Part model, mm, in its own coordinate system. A direction names the side the tool comes from. Round coordinates to 2 decimals unless told otherwise and drop trailing zeros. Order: outer loops, then holes, each group sorted by start corner. A loop starts at its lowest first (then second) coordinate and runs counter-clockwise, first axis right, second up. Notation, with made-up numbers: (9, 25) - (26, 25) arc R25 cw to (26, 43) - close; hole circle Ø4 at (70.25, 24). An arc over 180 degrees is marked (long way). Return JSON: item names as keys, results as strings. Group by question number.
Item 1: Saw through at B-B on y = 43. List the corners of the cut face in (x, z), and give its area (3 significant figures).
Item 2: Two-plate mould, pull along X, no slides. Class faces 5 (the face through (-46.04, 1.3, -17.45)), 6 (the face through (11, -11, -35)), 7 (the face through (-14.012, -41.154, -17.451)): released by +X, released by -X, zero draft, split by the parting line, or undercut.
Item 3: Probe probe 1 along Y at (x, z) = (-40, 17); probe 2 along X at (y, z) = (-5, -20.5); probe 3 along Y at (x, z) = (0, 1.5). List the from-to ranges inside material, lowest first.
Item 4: Saw through at D-D on z = 24.5. List the corners of the cut face in (x, y), and give its area (3 significant figures).
Item 5: Saw through at A-A on x = -40. List the corners of the cut face in (y, z), and give its area (3 significant figures).
Item 6: Drop flat-ended pins along their axis: pin 1 (6 mm diameter, centred on x = 152.5, z = 16, fed in from -Y); pin 2 (8 mm diameter, centred on x = -1, z = -0.5, fed in from +Y); pin 3 (13 mm diameter, centred on x = 15, y = -43, fed in from -Z); pin 4 (1.5 mm diameter, centred on x = 29.5, y = 2.5, fed in from +Z). Give the stop position or say it passes through.
Item 7: Tool access for faces 1 (the face through (-25, 9, 14)), 2 (the face through (226, 0, -6)), 3 (the face through (102.63, -9.45, 15.3)), 4 (the face through (102.185, 9.451, -15.413)): list every direction of +Z, -Z, +X, -X, +Y, -Y with a clear straight run to the whole face (end or side of a thin tool).
Item 8: Saw through at C-C on x = 250. List the corners of the cut face in (y, z).
```python
from build123d import *

# Parameters (mm, degrees)
SKETCH1_R           = 25.416099274
SKETCH1_R_2         = 15.345879333
BOSS_EXTRUDE3_DEPTH = 35
BOSS_EXTRUDE4_DEPTH = 21
CUT_EXTRUDE1_DEPTH  = 21
SKETCH1_7_R         = 17.5
SKETCH1_7_R_2       = 12
BOSS_EXTRUDE5_DEPTH = 21
BOSS_EXTRUDE6_START = 14
SKETCH1_8_R         = 5
BOSS_EXTRUDE6_DEPTH = 7
CUT_EXTRUDE2_DEPTH  = 18.5


with BuildPart() as part:
    # Sketch1 → Boss-Extrude3 (new body, symmetric)
    with BuildSketch(Plane.XY):
        Circle(SKETCH1_R)
        Circle(SKETCH1_R_2, mode=Mode.SUBTRACT)
    extrude(amount=BOSS_EXTRUDE3_DEPTH, both=True)

    # Sketch1<6> → Boss-Extrude4 (add, symmetric)
    with BuildSketch(Plane.XY):
        with BuildLine():
            ThreePointArc((234.99166898, -9), (232.5, 0), (234.99166898, 9))
            Line((234.99166898, 9), (87, 13))
            ThreePointArc((87, 13), (86.400314561, 13.01370903), (85.800764144, 13.032413604))
            Line((85.800764144, 13.032413604), (20.667586541, 14.792868853))
            ThreePointArc((20.667586541, 14.792868853), (24.199871215, 7.768161657), (25.416099274, 0))
            ThreePointArc((25.416099274, 0), (24.199871215, -7.768161657), (20.667586541, -14.792868853))
            Line((20.667586541, -14.792868853), (85.800764144, -13.032413604))
            ThreePointArc((85.800764144, -13.032413604), (86.400314561, -13.01370903), (87, -13))
            Line((87, -13), (234.99166898, -9))
        make_face()
    extrude(amount=BOSS_EXTRUDE4_DEPTH, both=True)

    # Sketch2 → Cut-Extrude1 (cut, symmetric)
    with BuildSketch(Plane(origin=(0, 0, 0), x_dir=(1, 0, 0), z_dir=(0, 1, 0))):
        with BuildLine():
            Line((118.656620919, 13.062509397), (234.99166898, 9))
            Line((234.99166898, 9), (234.99166898, 21))
            Line((234.99166898, 21), (87, 21))
            ThreePointArc((87, 21), (102.408517533, 15.35701958), (118.656620919, 13.062509397))
        make_face()
        with BuildLine():
            Line((87, -21), (234.99166898, -21))
            Line((234.99166898, -21), (234.99166898, -9))
            Line((234.99166898, -9), (118.656620919, -13.062509397))
            ThreePointArc((118.656620919, -13.062509397), (102.408517533, -15.35701958), (87, -21))
        make_face()
    extrude(amount=CUT_EXTRUDE1_DEPTH, both=True, mode=Mode.SUBTRACT)

    # Sketch1<7> → Boss-Extrude5 (add, symmetric)
    with BuildSketch(Plane.XY):
        with Locations((250, 0)):
            Circle(SKETCH1_7_R)
        with Locations((250, 0)):
            Circle(SKETCH1_7_R_2, mode=Mode.SUBTRACT)
    extrude(amount=BOSS_EXTRUDE5_DEPTH, both=True)

    # Sketch1<8> → Boss-Extrude6 (add)
    with BuildSketch(Plane.XY.offset(BOSS_EXTRUDE6_START)):
        with BuildLine():
            Line((20.667586541, 14.792868853), (85.800764144, 13.032413604))
            ThreePointArc((85.800764144, 13.032413604), (52.537254482, 22.523369258), (27.53882285, 46.431897657))
            ThreePointArc((27.53882285, 46.431897657), (18.775996279, 55.439527809), (6.484634563, 52.82285862))
            ThreePointArc((6.484634563, 52.82285862), (-13.863951623, 42.202436765), (-36.520978816, 38.525829777))
            ThreePointArc((-36.520978816, 38.525829777), (-51.292032009, 32.441274184), (-49.011059213, 16.629791258))
            ThreePointArc((-49.011059213, 16.629791258), (-46.024075038, 1.080135069), (-46.508202044, -14.746409188))
            ThreePointArc((-46.508202044, -14.746409188), (-51.333950201, -32.367226465), (-33.774741186, -37.412543656))
            ThreePointArc((-33.774741186, -37.412543656), (-13.740515927, -41.247010721), (4.414359967, -50.546139748))
            ThreePointArc((4.414359967, -50.546139748), (17.277164415, -55.799004736), (27.53882285, -46.431897657))
            ThreePointArc((27.53882285, -46.431897657), (52.537254482, -22.523369258), (85.800764144, -13.032413604))
            Line((85.800764144, -13.032413604), (20.667586541, -14.792868853))
            ThreePointArc((20.667586541, -14.792868853), (-25.416099274, 0), (20.667586541, 14.792868853))
        make_face()
        with Locations((15, -43)):
            Circle(SKETCH1_8_R, mode=Mode.SUBTRACT)
        with Locations((-40, -26)):
            Circle(SKETCH1_8_R, mode=Mode.SUBTRACT)
        with Locations((-40, 26)):
            Circle(SKETCH1_8_R, mode=Mode.SUBTRACT)
        with Locations((15, 43)):
            Circle(SKETCH1_8_R, mode=Mode.SUBTRACT)
    boss_extrude6 = extrude(amount=BOSS_EXTRUDE6_DEPTH)

    # Mirror1: Boss-Extrude6 across plane
    add(boss_extrude6.mirror(Plane.XY))

    # Sketch3 → Cut-Extrude2 (cut)
    with BuildSketch(Plane.XY.offset(21)):
        with BuildLine():
            Line((70, 6), (220, 6))
            ThreePointArc((220, 6), (226, 0), (220, -6))
            Line((220, -6), (70, -6))
            ThreePointArc((70, -6), (64, 0), (70, 6))
        make_face()
    cut_extrude2 = extrude(amount=-CUT_EXTRUDE2_DEPTH, mode=Mode.SUBTRACT)

    # Mirror2: Cut-Extrude2 across plane
    add(cut_extrude2.mirror(Plane.XY), mode=Mode.SUBTRACT)


solid = part.part
```
Filled in:
{
 "1": {"outline": "(-11.59, -21) - (10, -21) - (10, -14) - (-11.59, -14) - close; (-11.59, 14) - (10, 14) - (10, 21) - (-11.59, 21) - close; (20, -21) - (29.86, -21) - (29.86, -14) - (20, -14) - close; (20, 14) - (29.86, 14) - (29.86, 21) - (20, 21) - close", "area": "440 mm^2"},
 "2": {"face 5": "released by -X", "face 6": "zero draft", "face 7": "undercut"},
 "3": {"probe 1": "y = -39 to -31, -21 to 21, 31 to 39", "probe 2": "x = -45.8 to -14.51, 14.51 to 66.68, 233.23 to 239.09, 260.91 to 266.77", "probe 3": "y = -25.42 to -15.35, 15.35 to 25.42"},
 "4": {"outline": "circle Ø50.83 at (0, 0); hole circle Ø30.69 at (0, 0)", "area": "1,290 mm^2"},
 "5": {"outline": "(-39, -21) - (-31, -21) - (-31, -14) - (-39, -14) - close; (-39, 14) - (-31, 14) - (-31, 21) - (-39, 21) - close; (-21, -21) - (21, -21) - (21, -14) - (-21, -14) - close; (-21, 14) - (21, 14) - (21, 21) - (-21, 21) - close; (31, -21) - (39, -21) - (39, -14) - (31, -14) - close; (31, 14) - (39, 14) - (39, 21) - (31, 21) - close", "area": "812 mm^2"},
 "6": {"pin 1": "passes through", "pin 2": "stops at y = 25.42", "pin 3": "stops at z = -21", "pin 4": "stops at z = 21"},
 "7": {"face 1": "none", "face 2": "-Z", "face 3": "+Z, +Y, -Y", "face 4": "-Z, +Y, -Y"},
 "8": {"outline": "(-17.5, -21) - (-12, -21) - (-12, 21) - (-17.5, 21) - close; (12, -21) - (17.5, -21) - (17.5, 21) - (12, 21) - close"}
}
